```python
from build123d import *

# Parameters (mm, degrees)
EXTRUDE_1_DEPTH     = 10
SKETCH_2_R          = 0.79375
CUT_EXTRUDE_1_DEPTH = 18.320508076


with BuildPart() as part:
    # 草图1 → 凸台-拉伸1 (new body)
    with BuildSketch(Plane.XY):
        with BuildLine():
            Line((0, 4.7625), (0, 10))
            Line((0, 10), (-10, 10))
            Line((-10, 10), (-10, -10))
            Line((-10, -10), (0, -10))
            Line((0, -10), (0, -4.7625))
            ThreePointArc((0, -4.7625), (-4.7625, 0), (0, 4.7625))
        make_face()
    extrude(amount=EXTRUDE_1_DEPTH)

    # 草图2 → 切除-拉伸1 (cut, through all)
    with BuildSketch(Plane(origin=(0, 0, 0), x_dir=(0, 0, -1), z_dir=(1, 0, 0))):
        with Locations((-5, 7.38125)):
            Circle(SKETCH_2_R)
        with Locations((-4.222922478, -7.38125)):
            Circle(SKETCH_2_R)
    extrude(amount=-CUT_EXTRUDE_1_DEPTH, mode=Mode.SUBTRACT)


solid = part.part
```
Read the model definition and answer for the solid it produces. Units are mm, in the model's axes. Give positions to 0.01 mm unless a question says otherwise; leave off trailing zeros. Write each loop counter-clockwise with the first axis right and the second up, starting at its lowest first coordinate (ties: lowest second). Pieces come first, ordered by that corner, then holes. Notation, with made-up numbers: (11, -14.5) - (69, -14.5) arc R15 cw to (69, 8.5) - close; hole circle Ø7 at (72.5, -3.5). An arc over 180 degrees is marked (long way). Write item = value, one per line. Start each with the question number.
Item 1: Find section C-C (y = 0). Give the vertices of the cut face in (x, z), then the cut area to 3 significant figures.
Item 2: Find section A-A (x = -2). Give the vertices of the cut face in (y, z), then the cut area to 3 significant figures.
Item 3: Find the intervals of material crossed by probe 1 along Y at (x, z) = (-5, 4.5); probe 2 along Z at (x, y) = (-4.75, 7.75); probe 3 along Y at (x, z) = (-1, 9.25), in increasing order. Write a range as [from, to].
Item 4: Find section D-D (x = -1). Give the vertices of the cut face in (y, z).
Item 5: Each of these flat-tipped pins is pushed along its axis until it touches: P1, Ø6, axis at y = 3.5, z = 8.5, coming from the +X side; P2, Ø1.3, axis at y = 7.38, z = 5, coming from the -X side. Where does it stop, or does it pass through?
Item 6: The mould has two halves that part along Y. Classify faces 1 (the flat face through (-5, -10, 5)), 2 (the flat face through (0, -8, 5)), 3 (the cylindrical face through (-4.76, -0.1, 4.93)): +Y half, -Y half, draft (parallel to the pull), parting line (faces both ways), or undercut.
Item 7: Find section B-B (z = 4.5). Give the vertices of the cut face in (x, y) (1 decimal).
Response:
q1.outline = (-10, 0) - (-4.76, 0) - (-4.76, 10) - (-10, 10) - close
q1.area = 52.4 mm²
q2.outline = (-10, 0) - (-4.32, 0) - (-4.32, 10) - (-10, 10) - close; (4.32, 0) - (10, 0) - (10, 10) - (4.32, 10) - close; hole circle Ø1.59 at (-7.38, 4.22); hole circle Ø1.59 at (7.38, 5)
q2.area = 110 mm²
q3.probe_1 = [-10, -8.13], [-6.64, 6.76], [8, 10]
q3.probe_2 = [0, 4.3], [5.7, 10]
q3.probe_3 = [-10, -4.66], [4.66, 10]
q4.outline = (-10, 0) - (-4.66, 0) - (-4.66, 10) - (-10, 10) - close; (4.66, 0) - (10, 0) - (10, 10) - (4.66, 10) - close; hole circle Ø1.59 at (-7.38, 4.22); hole circle Ø1.59 at (7.38, 5)
q5.P1 = 0
q5.P2 = through
q6.face_1 = -Y half
q6.face_2 = draft
q6.face_3 = undercut
q7.outline = (-10, -10) - (0, -10) - (0, -8.1) - (-10, -8.1) - close; (-10, -6.6) - (0, -6.6) - (0, -4.8) arc R4.8 cw to (0, 4.8) - (0, 6.8) - (-10, 6.8) - close; (-10, 8) - (0, 8) - (0, 10) - (-10, 10) - close
